```python
from build123d import *

# Parameters (mm, degrees)
SKETCH1_W           = 55
SKETCH1_H           = 49
BOSS_EXTRUDE1_DEPTH = 2
SKETCH2_R           = 1.45
BOSS_EXTRUDE2_DEPTH = 10


with BuildPart() as part:
    # Sketch1 → Boss-Extrude1 (new body)
    with BuildSketch(Plane(origin=(0, 0, 0), x_dir=(1, 0, 0), z_dir=(0, 1, 0))):
        with Locations((27.5, 24.5)):
            Rectangle(SKETCH1_W, SKETCH1_H)
    extrude(amount=-BOSS_EXTRUDE1_DEPTH)

    # Sketch2 → Boss-Extrude2 (add)
    with BuildSketch(Plane(origin=(0, 0, 0), x_dir=(1, 0, 0), z_dir=(0, 1, 0))):
        with Locations((3.45, 3.45)):
            Circle(SKETCH2_R)
        with Locations((51.550000042, 3.45)):
            Circle(SKETCH2_R)
        with Locations((51.550000042, 45.55)):
            Circle(SKETCH2_R)
        with Locations((3.45, 45.55)):
            Circle(SKETCH2_R)
    extrude(amount=BOSS_EXTRUDE2_DEPTH)


solid = part.part
```
Geometry check sheet. Reference: the model listing, model coordinates, mm. A direction names the side the tool comes from. Round coordinates to 2 decimals unless told otherwise and drop trailing zeros. Order: outer loops, then holes, each group sorted by start corner. A loop starts at its lowest first (then second) coordinate and runs counter-clockwise, first axis right, second up. Notation, with made-up numbers: (-8.5, 87) - (-3.5, 87) arc R26 ccw to (-3.5, 107) - close; hole circle Ø8 at (-11.5, 48). An arc over 180 degrees is marked (long way). Use a Markdown table: item, result. Add a question column.
1) Section check C-C (y = 2). Record the cut outline in (x, z), then the cut area to 3 significant figures.
2) Set-up check for faces 1 (the flat face through (27, -2, -25)), 2 (the cylindrical face through (2.38, 4.93, -4.43)): record each of +Z, -Z, +X, -X, +Y, -Y from which the full face is reachable in a straight line by a thin tool's end or side.
3) Section check B-B (z = -45.55). Record the cut outline in (x, y).
4) Mould release check, pull along Z, two halves, no side actions. Record for faces 3 (the flat face through (0, -1, -24)), 4 (the flat face through (27, -1, -49)), 5 (the cylindrical face through (52.93, 4.93, -45.99)): released by +Z, released by -Z, zero draft, split by the parting line, or undercut.
5) Section check D-D (z = -30). Record the cut outline in (x, y), then the cut area to 3 significant figures.
6) Section check A-A (x = 3.45). Record the cut outline in (y, z), then the cut area to 3 significant figures.
7) Thickness scan on line 1 along Y through (x, z) = (5.5, -2.5); line 2 along X through (y, z) = (3, -45); line 3 along Z through (x, y) = (50.5, 3). Record the ranges inside material, lowest first.
8) Gauge pin test, flat ends, axial feed: P1, Ø6, axis at x = 13.5, z = -39.5, coming from the +Y side; P2, Ø3, axis at y = 7.5, z = -7, coming from the -X side. Record the tip position at first contact, or that the pin passes through.
Established:
| question | item | result |
|---|---|---|
| 1 | outline | circle Ø2.9 at (3.45, -45.55); circle Ø2.9 at (3.45, -3.45); circle Ø2.9 at (51.55, -45.55); circle Ø2.9 at (51.55, -3.45) |
| 1 | area | 26.4 mm2 |
| 2 | face 1 | +Z, -Z, +X, -X, -Y |
| 2 | face 2 | +Y |
| 3 | outline | (0, -2) - (55, -2) - (55, 0) - (53, 0) - (53, 10) - (50.1, 10) - (50.1, 0) - (4.9, 0) - (4.9, 10) - (2, 10) - (2, 0) - (0, 0) - close |
| 4 | face 3 | zero draft |
| 4 | face 4 | released by -Z |
| 4 | face 5 | undercut |
| 5 | outline | (0, -2) - (55, -2) - (55, 0) - (0, 0) - close |
| 5 | area | 110 mm2 |
| 6 | outline | (-2, -49) - (0, -49) - (0, -47) - (10, -47) - (10, -44.1) - (0, -44.1) - (0, -4.9) - (10, -4.9) - (10, -2) - (0, -2) - (0, 0) - (-2, 0) - close |
| 6 | area | 156 mm2 |
| 7 | line 1 | -2 to 0 |
| 7 | line 2 | 2.11 to 4.79, 50.21 to 52.89 |
| 7 | line 3 | -46.55 to -44.55, -4.45 to -2.45 |
| 8 | P1 | y = 0 |
| 8 | P2 | through |
